```python
from build123d import *
from OCP.BRepFilletAPI import BRepFilletAPI_MakeChamfer

# Parameters (mm, degrees)
SKETCH1_W            = 69.35
SKETCH1_H            = 113.5
BOSS_EXTRUDE5_DEPTH  = 2
SKETCH2_R            = 2.35
CUT_EXTRUDE3_DEPTH   = 2.5
FACE_CHAMFER_SIZE    = 1.5
FACE_CHAMFER_SIZE2   = 1.258649447
SKETCH4_W            = 60.238416088
SKETCH4_H            = 90.514495008
CUT_EXTRUDE6_DEPTH   = 0.5
SKETCH5_W            = 20.93325514
SKETCH5_H            = 17.0989254
SKETCH5_W_2          = 13.4
SKETCH5_H_2          = 10.2
BOSS_EXTRUDE7_DEPTH  = 4.5
SKETCH6_W            = 13.4
SKETCH6_H            = 10.2
CUT_EXTRUDE7_DEPTH   = 4.1
SKETCH7_W            = 20.93325514
SKETCH7_H            = 17.0989254
BOSS_EXTRUDE8_DEPTH  = 0.75
SKETCH8_W            = 2.621357244
SKETCH8_H            = 10.2
CUT_EXTRUDE8_DEPTH   = 0.5
SKETCH10_W           = 1.18316995
SKETCH10_H           = 0.660821766
BOSS_EXTRUDE11_DEPTH = 1
FILLET1_R            = 0.9
SKETCH11_W           = 4.263170706
SKETCH11_H           = 10.2
CUT_EXTRUDE9_DEPTH   = 10


with BuildPart() as part:
    # Sketch1 → Boss-Extrude5 (new body)
    with BuildSketch(Plane(origin=(0, 0, 0), x_dir=(1, 0, 0), z_dir=(0, 1, 0))):
        Rectangle(SKETCH1_W, SKETCH1_H)
    extrude(amount=BOSS_EXTRUDE5_DEPTH)

    # Sketch2 → Cut-Extrude3 (cut)
    with BuildSketch(Plane(origin=(0, 2, 0), x_dir=(1, 0, 0), z_dir=(0, 1, 0))):
        with Locations(Location((0, 41.476002696, 0), (0, 0, 270))):
            Circle(SKETCH2_R)
        with Locations(Location((0, -41.476002696, 0), (0, 0, 90))):
            Circle(SKETCH2_R)
    extrude(amount=-CUT_EXTRUDE3_DEPTH, mode=Mode.SUBTRACT)

    # face chamfer: one chamfer whose edges measure the first distance from different faces: ONE call of the kernel's chamfer builder (chamfer() names one face for all edges)
    face_chamfer_edges_1 = [part.edges().sort_by_distance(p)[0] for p in [
        (0, 2, -56.75),
        (-34.675, 2, 0),
        (0, 2, 56.75),
        (34.675, 2, 0),
    ]]
    face_chamfer_side_1 = [part.faces().sort_by_distance(p)[0] for p in [
        (0, 2, 0),
    ]]
    face_chamfer_edges_2 = [part.edges().sort_by_distance(p)[0] for p in [
        (0, 2, -43.826002696),
    ]]
    face_chamfer_side_2 = [part.faces().sort_by_distance(p)[0] for p in [
        (0, 1, -43.826002696),
    ]]
    face_chamfer_edges_3 = [part.edges().sort_by_distance(p)[0] for p in [
        (0, 2, 43.826002696),
    ]]
    face_chamfer_side_3 = [part.faces().sort_by_distance(p)[0] for p in [
        (0, 1, 43.826002696),
    ]]
    face_chamfer = BRepFilletAPI_MakeChamfer(part.part.solid().wrapped)
    for e in face_chamfer_edges_1:
        face_chamfer.Add(FACE_CHAMFER_SIZE, FACE_CHAMFER_SIZE2, e.wrapped, face_chamfer_side_1[0].wrapped)  # the first distance lies on this face
    for e in face_chamfer_edges_2:
        face_chamfer.Add(FACE_CHAMFER_SIZE, FACE_CHAMFER_SIZE2, e.wrapped, face_chamfer_side_2[0].wrapped)  # the first distance lies on this face
    for e in face_chamfer_edges_3:
        face_chamfer.Add(FACE_CHAMFER_SIZE, FACE_CHAMFER_SIZE2, e.wrapped, face_chamfer_side_3[0].wrapped)  # the first distance lies on this face
    add(Compound.cast(face_chamfer.Shape()), mode=Mode.REPLACE)

    # Sketch4 → Cut-Extrude6 (cut)
    with BuildSketch(Plane(origin=(0, 0, 0), x_dir=(-1, 0, 0), z_dir=(0, -1, 0))):
        Rectangle(SKETCH4_W, SKETCH4_H)
    extrude(amount=-CUT_EXTRUDE6_DEPTH, mode=Mode.SUBTRACT)

    # Sketch5 → Boss-Extrude7 (add)
    with BuildSketch(Plane(origin=(0, 2, 0), x_dir=(1, 0, 0), z_dir=(0, 1, 0))):
        Rectangle(SKETCH5_W, SKETCH5_H)
        Rectangle(SKETCH5_W_2, SKETCH5_H_2, mode=Mode.SUBTRACT)
    extrude(amount=-BOSS_EXTRUDE7_DEPTH)

    # Sketch6 → Cut-Extrude7 (cut)
    with BuildSketch(Plane(origin=(0, 2, 0), x_dir=(1, 0, 0), z_dir=(0, 1, 0))):
        Rectangle(SKETCH6_W, SKETCH6_H)
    extrude(amount=-CUT_EXTRUDE7_DEPTH, mode=Mode.SUBTRACT)

    # Sketch7 → Boss-Extrude8 (add)
    with BuildSketch(Plane.XZ.offset(2.5)):
        Rectangle(SKETCH7_W, SKETCH7_H)
    extrude(amount=BOSS_EXTRUDE8_DEPTH)

    # Sketch8 → Cut-Extrude8 (cut)
    with BuildSketch(Plane(origin=(0, -2.5, 0), x_dir=(1, 0, 0), z_dir=(0, 1, 0))):
        with Locations((-5.389321378, 0)):
            Rectangle(SKETCH8_W, SKETCH8_H)
    extrude(amount=-CUT_EXTRUDE8_DEPTH, mode=Mode.SUBTRACT)

    # Sketch10 → Boss-Extrude11 (add)
    with BuildSketch(Plane.ZY.offset(-6.7)):
        with Locations((-0.045919003, 0.630410883)):
            Rectangle(SKETCH10_W, SKETCH10_H)
    extrude(amount=BOSS_EXTRUDE11_DEPTH)

    # Fillet1
    # the kernel refuses this fillet: 0.9 mm, written as the material it takes off along each edge
    with BuildSketch(Plane(origin=(5.7, 0.960821766, 2.714758197), x_dir=(1, 0, 0), z_dir=(0, 0, -1))) as fillet1_piece_1:
        with BuildLine():
            CenterArc((0.86763689, 0.9), FILLET1_R, 195.411736224, 74.588263776)
            Line((0, 0.660821766), (-0.017352738, 0.656038202))
            ThreePointArc((-0.017352738, 0.656038202), (-0.018, 0.330410883), (-0.018, 0))
            Line((-0.018, 0), (0, -0.018))
            Line((0, -0.018), (0.86763689, -0.018))
            Line((0.86763689, -0.018), (0.86763689, 0))
        make_face()
    extrude(amount=5.521354399, mode=Mode.SUBTRACT)

    # Sketch11 → Cut-Extrude9 (cut)
    with BuildSketch(Plane(origin=(0, -3.25, 0), x_dir=(-1, 0, 0), z_dir=(0, -1, 0))):
        with Locations((4.568414647, 0)):
            Rectangle(SKETCH11_W, SKETCH11_H)
    extrude(amount=-CUT_EXTRUDE9_DEPTH, mode=Mode.SUBTRACT)


solid = part.part
```
For this review, take the finished solid that the model builds, in its own axes (mm). A direction names the side the tool comes from. Give positions to 0.01 mm unless a question says otherwise; leave off trailing zeros. Write each loop counter-clockwise with the first axis right and the second up, starting at its lowest first coordinate (ties: lowest second). Pieces come first, ordered by that corner, then holes. Notation, with made-up numbers: M 72.5,28 L 87.5,28 A30 cw 87.5,62 Z; hole C -39.75,-25 d8. An arc over 180 degrees is marked long. Answer as CSV lines item,"result".
1. For faces 4 (the flat face through (0, -1, -5.1)), 5 (the flat face through (7, 2, -1)), list the 3-axis set-ups (+Z, -Z, +X, -X, +Y, -Y) from which the entire face can be reached by the end or side of a thin tool; tool diameter is ignored.
Findings:
face 4,"+Y"
face 5,"+Z, -Z, +X, -X, +Y"
2. For pin 1 (0.8 mm diameter, centred on y = -3, z = -0.5, fed in from -X); pin 2 (2 mm diameter, centred on y = -0.5, z = -0.5, fed in from -X) (3 decimals); pin 3 (5 mm diameter, centred on x = 13, z = -10, fed in from -Y); pin 4 (1.5 mm diameter, centred on x = -6.5, y = -2, fed in from -Z), all flat-tipped, find the tip position at first contact; note any pin that passes through.
Findings:
pin 1,"stops at x = -10.47"
pin 2,"stops at x = -34.675"
pin 3,"stops at y = 0.5"
pin 4,"stops at z = -8.55"
3. Draft analysis for pull direction X (two halves, no side actions). For faces 1 (the flat face through (-6.7, -1, 0)), 2 (the flat face through (6.7, 0, 0)), 3 (the flat face through (0, -3.25, 0)), state which applies: +X half, -X half, draft (parallel to the pull), parting line (faces both ways), or undercut.
Findings:
face 1,"undercut"
face 2,"undercut"
face 3,"draft"
4. Consider section B-B, the plane x = 0. Write out the cut boundary in (y, z), then the cut area to 3 significant figures.
Findings:
outline,"M -3.25,-8.55 L 0.5,-8.55 L 0.5,-39.13 L 2,-37.87 L 2,-5.1 L -2.5,-5.1 L -2.5,5.1 L 2,5.1 L 2,37.87 L 0.5,39.13 L 0.5,8.55 L -3.25,8.55 Z; M 0,-56.75 L 0.74,-56.75 L 2,-55.25 L 2,-45.08 L 0.5,-43.83 L 0.5,-45.26 L 0,-45.26 Z; M 0,45.26 L 0.5,45.26 L 0.5,43.83 L 2,45.08 L 2,55.25 L 0.74,56.75 L 0,56.75 Z"
area,"180 mm2"
5. Consider section D-D, the plane x = 12.5. Write out the cut boundary in (y, z).
Findings:
outline,"M 0,-56.75 L 0.74,-56.75 L 2,-55.25 L 2,55.25 L 0.74,56.75 L 0,56.75 L 0,45.26 L 0.5,45.26 L 0.5,-45.26 L 0,-45.26 Z"
6. Wall thickness on line 1 (X direction, y = -1.2, z = -2); line 2 (Z direction, x = -5, y = -2.6); line 3 (Z direction, x = 6, y = 0.7): over which ranges is each line inside the solid? List them lowest first.
Findings:
line 1,"x = -10.47 to -6.7, 6.7 to 10.47"
line 2,"z = -8.55 to -5.1, 5.1 to 8.55"
line 3,"z = -56.75 to -5.1, -0.64 to 0.55, 5.1 to 56.75"
7. Consider section C-C, the plane z = -36. Write out the cut boundary in (x, y) (3 decimals), then the cut area to 3 significant figures.
Findings:
outline,"M -34.675,0 L -30.119,0 L -30.119,0.5 L 30.119,0.5 L 30.119,0 L 34.675,0 L 34.675,0.741 L 33.175,2 L -33.175,2 L -34.675,0.741 Z"
area,"107 mm2"
8. Consider section A-A, the plane y = -0.85. Write out the cut boundary in (x, z), then the cut area to 3 significant figures.
Findings:
outline,"M -10.47,-8.55 L 10.47,-8.55 L 10.47,8.55 L -10.47,8.55 Z; hole M -6.7,-5.1 L 6.7,-5.1 L 6.7,5.1 L -6.7,5.1 Z"
area,"221 mm2"
